Job drawing, mm, ordinate dimensions from the low corner. One solid piece. Coordinates: 2 decimals unless noted, no trailing zeros. Order: outer loops, then holes, each group sorted by start corner. A loop starts at its lowest first (then second) coordinate and runs counter-clockwise, first axis right, second up. Notation, with made-up numbers: M -9.5,-37.75 L 48.5,-37.75 A17 cw 48.5,-10.75 Z; hole C 55.25,-15.5 d8. An arc over 180 degrees is marked long. Write item = value, one per line. Start each with the question number.
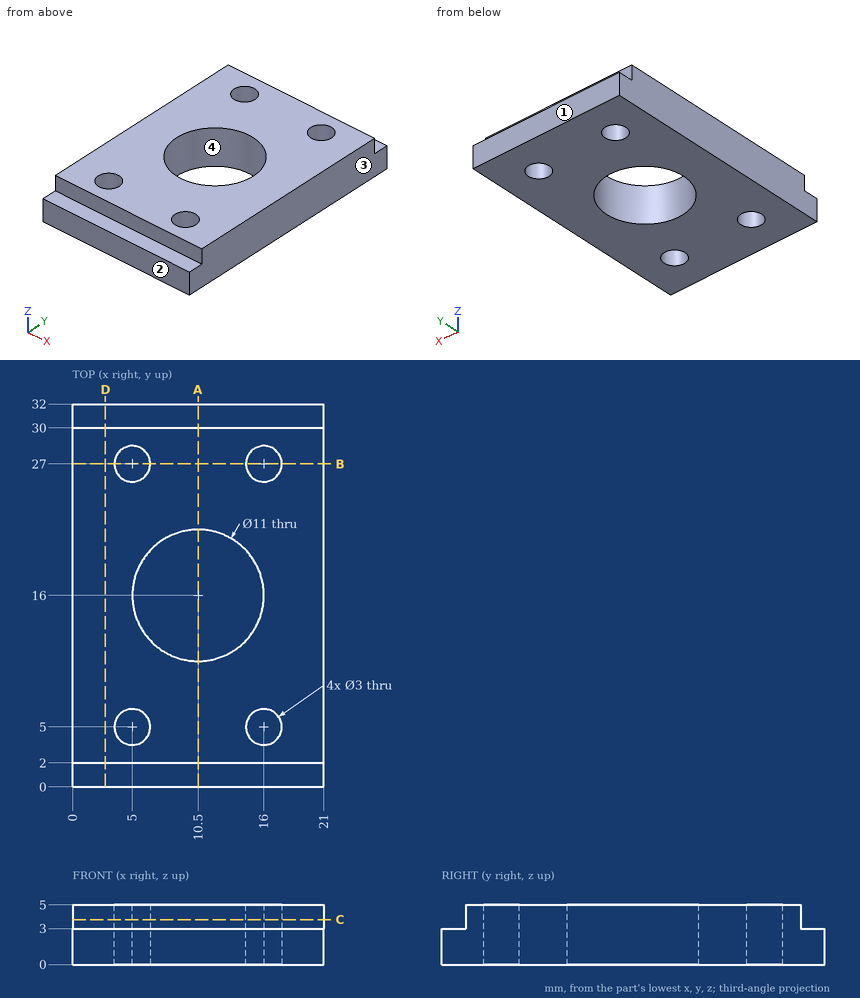
Item 1: Cut at D-D, the plane x = 2.75. Write the cut outline in (y, z), and give its area (3 significant figures).
Item 2: Flat gauge pins, fed straight in: pin 1 (2.5 mm diameter, centred on x = 16, y = 5, fed in from -Z); pin 2 (1.6 mm diameter, centred on x = 10, z = 4, fed in from +Y); pin 3 (0.6 mm diameter, centred on x = 9, y = 30.5, fed in from +Z); pin 4 (1.6 mm diameter, centred on x = 11.5, z = 4, fed in from -Y). Where does each tip first touch, or does it go through?
Item 3: Cut at B-B, the plane y = 27. Write the cut outline in (x, z).
Item 4: Pull direction Y, two halves, no side cores. Call the marked faces 1, 2, 3 and 4: pulls with the +Y half, pulls with the -Y half, needs draft (parallel to the pull), parting line crosses it, or undercut.
Item 5: Wall check: line 1 along Y through (x, z) = (10.5, 3.3); line 2 along X through (y, z) = (28, 4.5); line 3 along X through (y, z) = (5.5, 0.8). Give the ranges that are in metal, low to high. Write a range as [from, to].
Item 6: Cut at A-A, the plane x = 10.5. Write the cut outline in (y, z).
Item 7: Cut at C-C, the plane z = 3.75. Write the cut outline in (x, y), and give its area (3 significant figures).
Filled sheet:
q1.outline = M 0,0 L 32,0 L 32,3 L 30,3 L 30,5 L 2,5 L 2,3 L 0,3 Z
q1.area = 152 mm2
q2.pin_1 = through
q2.pin_2 = 30
q2.pin_3 = 3
q2.pin_4 = 2
q3.outline = M 0,0 L 3.5,0 L 3.5,5 L 0,5 Z; M 6.5,0 L 14.5,0 L 14.5,5 L 6.5,5 Z; M 17.5,0 L 21,0 L 21,5 L 17.5,5 Z
q4.face_1 = pulls with the +Y half
q4.face_2 = pulls with the -Y half
q4.face_3 = needs draft
q4.face_4 = undercut
q5.line_1 = [2, 10.5], [21.5, 30]
q5.line_2 = [0, 3.88], [6.12, 14.88], [17.12, 21]
q5.line_3 = [0, 3.59], [6.41, 14.59], [17.41, 21]
q6.outline = M 0,0 L 10.5,0 L 10.5,5 L 2,5 L 2,3 L 0,3 Z; M 21.5,0 L 32,0 L 32,3 L 30,3 L 30,5 L 21.5,5 Z
q7.outline = M 0,2 L 21,2 L 21,30 L 0,30 Z; hole C 5,5 d3; hole C 5,27 d3; hole C 10.5,16 d11; hole C 16,5 d3; hole C 16,27 d3
q7.area = 465 mm2
